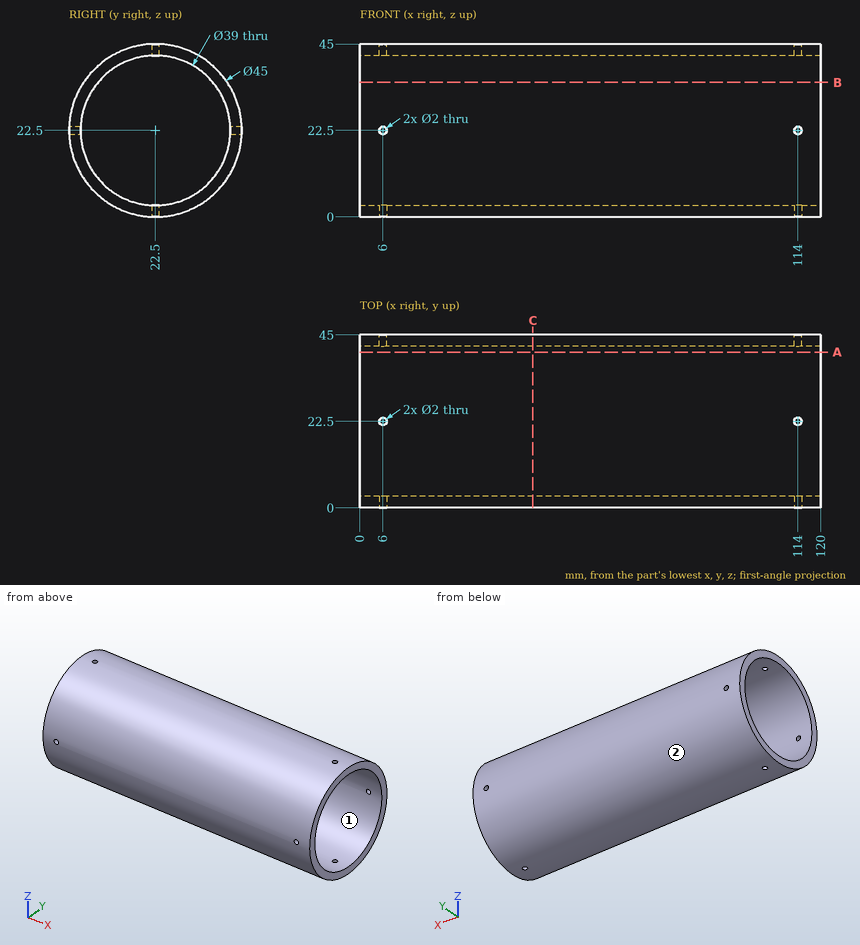
For this review, use the dimensioned drawing (mm, ordinates from the lowest corner) and the shaded views. Coordinates: 2 decimals unless noted, no trailing zeros. Order: outer loops, then holes, each group sorted by start corner. A loop starts at its lowest first (then second) coordinate and runs counter-clockwise, first axis right, second up. Notation, with made-up numbers: (0.25, -20) -> (51.25, -20) arc R14 cw to (51.25, -12) -> close; hole circle Ø2 at (30, -21). An arc over 180 degrees is marked (long way). One line per item, written item: value. Start each with the question number.
Q1. Take a section at B-B, the plane z = 35. State the section outline as (x, y) points, then the cut area to 3 significant figures.
Q2. Mouldability with a two-part tool opening along Z and no side actions: class the marked faces 1 and 2 as pulls with the +Z half, pulls with the -Z half, needs draft (parallel to the pull), parting line crosses it, or undercut.
Q3. Insertion check: pin 1 Ø5 at (x, y) = (94, 34) entering from +Z; pin 2 Ø1.5 at (x, z) = (27, 33) entering from +Y; pin 3 Ø8 at (x, z) = (34.5, 11.5) entering from -Y. Each pin has a flat end and moves straight along its axis. Give the tip position at first contact, or say it passes through.
Q4. For probe 1 along X at (y, z) = (1.1, 22.5); probe 2 along Z at (x, y) = (57, 22); probe 3 along Y at (x, z) = (14.5, 21.5), list the stretches that pass through material, from the lowest coordinate up.
Q5. Take a section at C-C, the plane x = 45. State the section outline as (y, z) points.
Q6. Take a section at A-A, the plane y = 40.5. State the section outline as (x, z) points.
Values follow:
1. outline: (0, 3.79) -> (120, 3.79) -> (120, 7.53) -> (0, 7.53) -> close; (0, 37.47) -> (120, 37.47) -> (120, 41.21) -> (0, 41.21) -> close
1. area: 898 mm2
2. face 1: undercut
2. face 2: parting line crosses it
3. pin 1: stops at z = 43.12
3. pin 2: stops at y = 42.78
3. pin 3: stops at y = 1.12
4. probe 1: x = 0 to 5, 7 to 113, 115 to 120
4. probe 2: z = 0.01 to 3.01, 41.99 to 44.99
4. probe 3: y = 0.02 to 3.03, 41.97 to 44.98
5. outline: circle Ø45 at (22.5, 22.5); hole circle Ø39 at (22.5, 22.5)
6. outline: (0, 9) -> (120, 9) -> (120, 15) -> (0, 15) -> close; (0, 30) -> (120, 30) -> (120, 36) -> (0, 36) -> close
